Design review of the part built by this model. Coordinates are the model's own, in mm. Face numbers are marked on the shaded views. A direction names the side the tool comes from. Round coordinates to 2 decimals unless told otherwise and drop trailing zeros. Write each loop counter-clockwise with the first axis right and the second up, starting at its lowest first coordinate (ties: lowest second). Pieces come first, ordered by that corner, then holes.
from build123d import *

# Parameters (mm, degrees)
F1_DEPTH = 25.4
F2_R     = 5.08
F3_R     = 5.08
F5_D     = 12.7


with BuildPart() as f1:
    # F0 (on Front) → F1 (new body)
    with BuildSketch(Plane.XZ):
        Polygon((0, 12.7), (0, 0), (31.75, 0), (31.75, 25.4), (19.05, 25.4), (19.05, 12.7), align=None)
    extrude(amount=F1_DEPTH)

    # F2
    f2_edges = [f1.edges().sort_by_distance(p)[0] for p in [
        (0, -25.4, 6.35),
    ]]
    fillet(f2_edges, radius=F2_R)

    # F3
    f3_edges = [f1.edges().sort_by_distance(p)[0] for p in [
        (0, 0, 6.35),
    ]]
    fillet(f3_edges, radius=F3_R)

    # F5 (through all)
    with Locations(Plane.XY.offset(12.7)):
        with Locations((9.731116, -12.168982)):
            Hole(F5_D / 2)

    # F6: F1 across face


with BuildPart() as f1_1:
    add(f1.part)
    add(f1.part.mirror(Plane(origin=(31.75, -12.7, 12.7), x_dir=(0, 1, 0), z_dir=(1, 0, 0))))


solid = f1_1.part
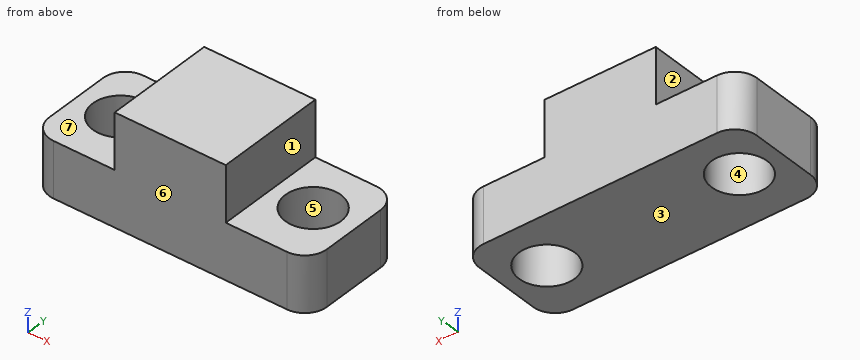
1) For line 1 along X through (y, z) = (-8.75, 4.5); line 2 along X through (y, z) = (-21, 17.5); line 3 along Z through (x, y) = (19, -2.25), list the stretches that pass through material, from the lowest coordinate up.
2) For P1, Ø2, axis at x = 14, y = -4.5, coming from the +Z side; P2, Ø6.5, axis at y = -7.5, z = 16, coming from the -X side; P3, Ø10, axis at x = 56, y = -5, coming from the -Z side; P4, Ø3, axis at y = -22, z = 20, coming from the +X side, all flat-tipped, find the tip position at first contact; note any pin that passes through.
3) The part is to be moulded in two halves that separate along Y. For the marked faces 4, 5, 6 and 7, say which applies: pulls with the +Y half, pulls with the -Y half, needs draft (parallel to the pull), parting line crosses it, or undercut.
4) For the marked faces 1, 2 and 3, list the 3-axis set-ups (+Z, -Z, +X, -X, +Y, -Y) from which the entire face can be reached by the end or side of a thin tool; tool diameter is ignored.
5) Add section C-C on z = 12. State the section outline as (x, y) points, and give its area (3 significant figures).
6) Add section B-B on y = -10.75. State the section outline as (x, z) points, and give its area (3 significant figures).
7) Add section D-D on x = 48.5. State the section outline as (y, z) points.
8) Add section A-A on x = 55. State the section outline as (y, z) points, and give its area (3 significant figures).
Computed:
1. line 1: x = 0 to 4.38, 15.08 to 48.42, 59.12 to 63.5
1. line 2: x = 19.05 to 44.45
1. line 3: z = 0 to 12.7
2. P1: stops at z = 12.7
2. P2: stops at x = 19.05
2. P3: stops at z = 0
2. P4: stops at x = 44.45
3. face 4: undercut
3. face 5: undercut
3. face 6: pulls with the -Y half
3. face 7: needs draft
4. face 1: +Z, +X, +Y, -Y
4. face 2: +Z, -X, +Y, -Y
4. face 3: -Z, +X, -X, +Y, -Y
5. outline: (0, -20.32) arc R5.08 ccw to (5.08, -25.4) - (58.42, -25.4) arc R5.08 ccw to (63.5, -20.32) - (63.5, -5.08) arc R5.08 ccw to (58.42, 0) - (5.08, 0) arc R5.08 ccw to (0, -5.08) - close; hole circle Ø12.7 at (9.73, -12.17); hole circle Ø12.7 at (53.77, -12.17)
5. area: 1,340 mm2
6. outline: (0, 0) - (3.54, 0) - (3.54, 12.7) - (0, 12.7) - close; (15.92, 0) - (47.58, 0) - (47.58, 12.7) - (44.45, 12.7) - (44.45, 25.4) - (19.05, 25.4) - (19.05, 12.7) - (15.92, 12.7) - close; (59.96, 0) - (63.5, 0) - (63.5, 12.7) - (59.96, 12.7) - close
6. area: 815 mm2
7. outline: (-25.4, 0) - (-15.71, 0) - (-15.71, 12.7) - (-25.4, 12.7) - close; (-8.62, 0) - (0, 0) - (0, 12.7) - (-8.62, 12.7) - close
8. outline: (-25.4, 0) - (-18.4, 0) - (-18.4, 12.7) - (-25.4, 12.7) - close; (-5.94, 0) - (0, 0) - (0, 12.7) - (-5.94, 12.7) - close
8. area: 164 mm2
